Geometry check sheet. Reference: the model listing, model coordinates, mm. Face numbers are marked on the shaded views. A direction names the side the tool comes from. Round coordinates to 2 decimals unless told otherwise and drop trailing zeros. Order: outer loops, then holes, each group sorted by start corner. A loop starts at its lowest first (then second) coordinate and runs counter-clockwise, first axis right, second up. Notation, with made-up numbers: (58, 89) -> (106, 89) arc R27 ccw to (106, 109) -> close; hole circle Ø8 at (22.5, 26.5). An arc over 180 degrees is marked (long way). Answer as a JSON object with one key per item and string values. Group by question number.
Autodesk Inventor part; units mm, degrees
ref_plane "YZ Plane" through (0, 0, 0) normal (1, 0, 0) x (0, 1, 0)
ref_plane "XZ Plane" through (0, 0, 0) normal (0, 1, 0) x (-1, 0, 0)
ref_plane "XY Plane" through (0, 0, 0) normal (0, 0, 1) x (1, 0, 0)
sketch "Sketch1" plane through (0, 0, 0) normal (0, 1, 0) x (-1, 0, 0)
  circle A0 centre (0, 0) radius 31
  dimension "d0" = 62
extrude "Extrusion1" add sketch "Sketch1" along normal blind 5
sketch "Sketch2" plane through (0, 5, 0) normal (0, 1, 0) x (1, 0, 0)
  circle A0 centre (0, 0) radius 20
  dimension "d3" = 40
extrude "Extrusion2" cut sketch "Sketch2" against normal blind 2
chamfer "Chamfer1" distance 2 angle 45 1 edges at (-20, 3, 0)
sketch "Sketch3" plane through (0, 0, 0) normal (0, -1, 0) x (1, 0, 0)
  line L0 (13.2, 13.2) -> (-13.2, 13.2)
  line L1 (-13.2, 13.2) -> (-13.2, -13.2)
  line L2 (-13.2, -13.2) -> (13.2, -13.2)
  line L3 (13.2, -13.2) -> (13.2, 13.2)
  point P0 (0, 0)
  dimension "d9" = 26.4
  dimension "d10" = 26.4
extrude "Extrusion3" cut sketch "Sketch3" against normal blind 6
sketch "Sketch4" plane through (0, 5, 0) normal (0, 1, 0) x (1, 0, 0)
  circle A0 centre (0, 16.2) radius 2
  circle A1 centre (0, -16.2) radius 2
  point P0 (0, 0)
  dimension "d13" = 4
  dimension "d14" = 4
extrude "Extrusion4" cut sketch "Sketch4" against normal blind 6
sketch "Sketch5" plane through (0, 0, 0) normal (0, -1, 0) x (1, 0, 0)
  line L0 (-13.2, -13.2) -> (-13.2, 13.2)
  line L1 (-13.2, 10) -> (-18.2, 10)
  line L2 (-18.2, 10) -> (-18.2, -10)
  line L3 (-18.2, -10) -> (-13.2, -10)
  line L4 (-13.2, -10) -> (-13.2, 10)
  line L5 (13.2, 13.2) -> (13.2, -13.2)
  line L6 (13.2, -10) -> (18.2, -10)
  line L7 (18.2, -10) -> (18.2, 10)
  line L8 (18.2, 10) -> (13.2, 10)
  line L9 (13.2, 10) -> (13.2, -10)
  point P0 (0, 0)
  dimension "d17" = 5
  dimension "d18" = 20
  dimension "d19" = 5
  dimension "d20" = 20
extrude "Extrusion5" add sketch "Sketch5" along normal blind 25.6
fillet "Fillet1" radius 10 4 edges at (15.7, -25.6, 10) (15.7, -25.6, -10) (-15.7, -25.6, -10) (-15.7, -25.6, 10)
fillet "Fillet2" radius 2 7 edges at (31, 0, 0) (18.2, -7.8001, 10) (18.2, -7.8001, -10) (18.2, -22.6711, 7.0711) (-18.2, -7.8001, -10) (-18.2, -7.8001, 10) (-18.2, -22.6711, -7.0711)
sketch "Sketch6" plane through (-18.2, 0, -8) normal (-1, 0, 0) x (0, 0, 1)
  circle A0 centre (8, -15.6) radius 2
  line L0 (0, 0) -> (16, 0)
  point P0 (8, 0)
  dimension "d25" = 4
  dimension "d31" = 15.6
extrude "Extrusion6" cut sketch "Sketch6" against normal blind 50
chamfer "Chamfer2" distance 2 angle 45 1 edges at (31, 5, 0)
properties part number "bigSpringMountB"
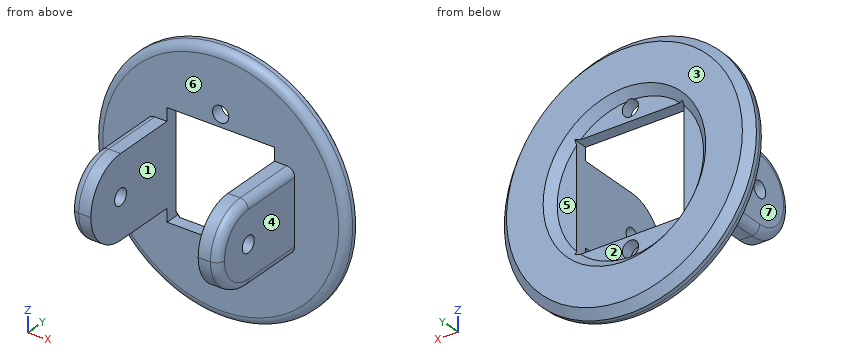
Item 1: Sectioned sample at B-B, the plane y = -9. Enter the section's corners in (x, z), then the cut area to 3 significant figures.
Item 2: Mould release check, pull along X, two halves, no side actions. Record for the marked faces 4, 5, 6 and 7: pulls with the +X half, pulls with the -X half, needs draft (parallel to the pull), parting line crosses it, or undercut.
Item 3: Depth check by flat-ended pin: pin 1 Ø1.5 at (x, y) = (-14.5, -11.5) entering from +Z; pin 2 Ø8 at (y, z) = (-15.5, 1) entering from -X; pin 3 Ø1.4 at (x, z) = (4.5, -16) entering from +Y; pin 4 Ø1.4 at (x, z) = (-0.5, 15.5) entering from +Y. Enter the tip coordinate at first touch or a pass-through.
Item 4: Set-up check for the marked faces 1, 2 and 3: record each of +Z, -Z, +X, -X, +Y, -Y from which the full face is reachable in a straight line by a thin tool's end or side.
Item 5: Thickness scan on L1, parallel to Z at x = 0, y = 2; L2, parallel to Z at x = 0, y = 1.45; L3, parallel to Y at x = -16, z = 0. Record the ranges inside material, lowest first.
Item 6: Sectioned sample at A-A, the plane x = 0. Count the separate pieces of the cut face and the enclosed holes in it, then the cut area to 3 significant figures.
Result:
{
 "1": {"outline": "(-18.2, -8) arc R2 ccw to (-16.2, -10) -> (-13.2, -10) -> (-13.2, 10) -> (-16.2, 10) arc R2 ccw to (-18.2, 8) -> close; (13.2, -10) -> (16.2, -10) arc R2 ccw to (18.2, -8) -> (18.2, 8) arc R2 ccw to (16.2, 10) -> (13.2, 10) -> close", "area": "197 mm2"},
 "2": {"face 4": "pulls with the +X half", "face 5": "undercut", "face 6": "needs draft", "face 7": "pulls with the -X half"},
 "3": {"pin 1": "stops at z = 10", "pin 2": "stops at x = -18.2", "pin 3": "stops at y = 3", "pin 4": "passes through"},
 "4": {"face 1": "+Y, -Y", "face 2": "+Y", "face 3": "+Z, -Z, +X, -X, +Y"},
 "5": {"L1": "z = -31 to -18.2, -14.2 to -13.2, 13.2 to 14.2, 18.2 to 31", "L2": "z = -30.92 to -18.2, -14.2 to -13.2, 13.2 to 14.2, 18.2 to 30.92", "L3": "y = -25.6 to -17.6, -13.6 to 3"},
 "6": {"separate pieces": "4", "enclosed holes": "0", "area": "125 mm2"}
}
